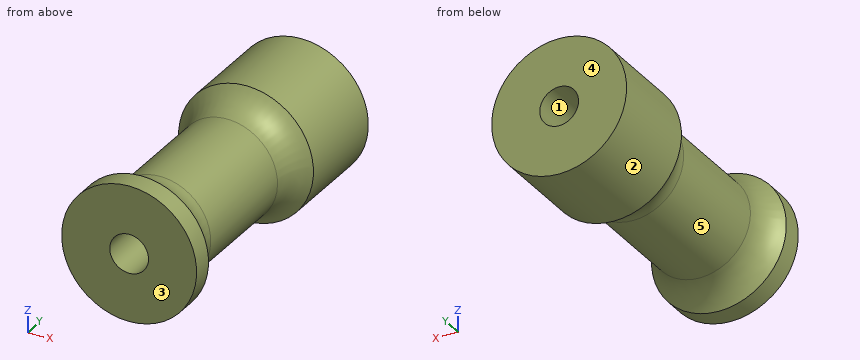
from build123d import *

# Parameters (mm, degrees)
FILLET_1_R = 5


with BuildPart() as part:
    # Эскиз1 → Повернуть1 (revolve)
    with BuildSketch(Plane.XY, mode=Mode.PRIVATE) as revolve_1_sk:
        Polygon((2.3, 0), (2.3, 36), (7.5, 36), (8, 36), (8, 24.5), (6, 24.5), (6, 2.5), (8, 2.5), (8, 0), (6, 0), align=None)
    revolve(revolve_1_sk.sketch.rotate(Axis((0, 0, 0), (0, 1, 0)), 90), axis=Axis((0, 0, 0), (0, 1, 0)))

    # Скругление1
    # the kernel refuses this fillet: 5 mm, written as the material it adds along each edge
    with BuildSketch(Plane(origin=(0, 2.5, 0), x_dir=(0, 0, -1), z_dir=(1, 0, 0))) as fillet_1_piece_1:
        with BuildLine():
            CenterArc((11, 4), FILLET_1_R, 180, 53.130102354)
            Line((8, 0), (7.94, -0.08))
            ThreePointArc((7.94, -0.08), (7, -0.1), (6, -0.1))
            Line((6, -0.1), (5.9, 0))
            Line((5.9, 0), (5.9, 4))
            Line((5.9, 4), (6, 4))
        make_face()
    revolve(axis=Axis((0, 2.5, 0), (0, 1, 0)))
    with BuildSketch(Plane(origin=(0, 24.5, 0), x_dir=(0, 0, -1), z_dir=(1, 0, 0))) as fillet_1_piece_2:
        with BuildLine():
            CenterArc((11, -4), FILLET_1_R, 126.869897646, 53.130102354)
            Line((6, -4), (5.9, -4))
            Line((5.9, -4), (5.9, 0))
            Line((5.9, 0), (6, 0.1))
            ThreePointArc((6, 0.1), (7, 0.1), (7.94, 0.08))
            Line((7.94, 0.08), (8, 0))
        make_face()
    revolve(axis=Axis((0, 24.5, 0), (0, 1, 0)))


solid = part.part
Verification items for the finished model (mm, model axes). Face numbers are marked on the shaded views. A direction names the side the tool comes from. Coordinates: 2 decimals unless noted, no trailing zeros. Write each loop counter-clockwise with the first axis right and the second up, starting at its lowest first coordinate (ties: lowest second). Pieces come first, ordered by that corner, then holes. Notation, with made-up numbers: (63.25, 83.5) - (80.25, 83.5) arc R23 cw to (80.25, 107.5) - close; hole circle Ø6 at (-18, -17). An arc over 180 degrees is marked (long way). Answer as a JSON object with one key per item and string values.
(1) Gauge pin test, flat ends, axial feed: pin 1 Ø6 at (y, z) = (5.5, 4) entering from -X; pin 2 Ø3 at (y, z) = (12.5, 4.5) entering from -X; pin 3 Ø6 at (y, z) = (6, 4) entering from +X. Record the tip position at first contact, or that the pin passes through.
Report:
{"pin 1": "x = -7.18", "pin 2": "x = -5.2", "pin 3": "x = 6.63"}
(2) Cross-section at A-A on x = 0. Record the cut outline in (y, z).
Report:
{"outline": "(0, -8) - (2.5, -8) arc R5 cw to (6.5, -6) - (20.5, -6) arc R5 cw to (24.5, -8) - (36, -8) - (36, -2.3) - (0, -2.3) - close; (0, 2.3) - (36, 2.3) - (36, 8) - (24.5, 8) arc R5 cw to (20.5, 6) - (6.5, 6) arc R5 cw to (2.5, 8) - (0, 8) - close"}
(3) Mould release check, pull along Z, two halves, no side actions. Record for the marked faces 1, 2 and 3: pulls with the +Z half, pulls with the -Z half, needs draft (parallel to the pull), parting line crosses it, or undercut.
Report:
{"face 1": "undercut", "face 2": "parting line crosses it", "face 3": "needs draft"}
(4) Cross-section at B-B on z = 0. Record the cut outline in (x, y).
Report:
{"outline": "(-8, 0) - (-2.3, 0) - (-2.3, 36) - (-8, 36) - (-8, 24.5) arc R5 cw to (-6, 20.5) - (-6, 6.5) arc R5 cw to (-8, 2.5) - close; (2.3, 0) - (8, 0) - (8, 2.5) arc R5 cw to (6, 6.5) - (6, 20.5) arc R5 cw to (8, 24.5) - (8, 36) - (2.3, 36) - close"}
(5) Cross-section at D-D on y = 25. Record the cut outline in (x, z).
Report:
{"outline": "circle Ø16 at (0, 0); hole circle Ø4.6 at (0, 0)"}
(6) Tool access check on the marked faces 4 and 5. Record the directions out of +Z, -Z, +X, -X, +Y, -Y that give a thin tool (end or side, any length) a straight path to the whole face; none if there is none.
Report:
{"face 4": "+Z, -Z, +X, -X, +Y", "face 5": "none"}
(7) Thickness scan on line 1 along X through (y, z) = (26.5, 0); line 2 along Z through (x, y) = (-0.5, 30) (3 decimals); line 3 along Y through (x, z) = (7.75, 0.25). Record the ranges inside material, lowest first.
Report:
{"line 1": "-8 to -2.3, 2.3 to 8", "line 2": "-7.984 to -2.245, 2.245 to 7.984", "line 3": "0 to 2.7, 24.3 to 36"}
(8) Cross-section at C-C on y = 13.5. Record the cut outline in (x, z).
Report:
{"outline": "circle Ø12 at (0, 0); hole circle Ø4.6 at (0, 0)"}
